Geometry: final body of the model. Coordinates: model frame, mm. Face numbers are marked on the shaded views. Round coordinates to 2 decimals unless told otherwise and drop trailing zeros. Order: outer loops, then holes, each group sorted by start corner. A loop starts at its lowest first (then second) coordinate and runs counter-clockwise, first axis right, second up. Notation, with made-up numbers: (19, 12.5) -> (48, 12.5) arc R9 ccw to (48, 18.5) -> close; hole circle Ø6 at (85, -13.75). An arc over 180 degrees is marked (long way). Put each result on its own line as item: value.
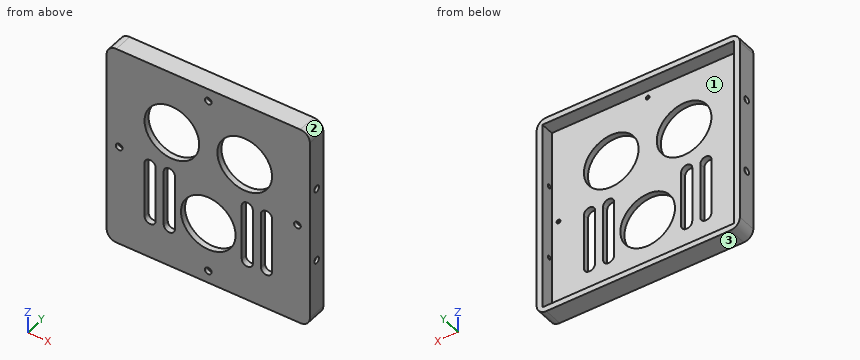
```python
from build123d import *

# Parameters (mm, degrees)
SKETCH1_W           = 106
SKETCH1_H           = 106
BOSS_EXTRUDE1_DEPTH = 10
SKETCH3_W           = 100
SKETCH3_H           = 100
CUT_EXTRUDE5_DEPTH  = 7
SKETCH7_R           = 14.25
CUT_EXTRUDE6_DEPTH  = 7
SKETCH9_R           = 1.75
CUT_EXTRUDE7_DEPTH  = 2
SKETCH11_R          = 1
CUT_EXTRUDE8_DEPTH  = 17
CUT_EXTRUDE9_DEPTH  = 1.5
SKETCH14_R          = 1
CUT_EXTRUDE10_DEPTH = 115.5
CUT_EXTRUDE11_START = -1.5
SKETCH15_R          = 1.75
CUT_EXTRUDE11_DEPTH = 1.5
FILLET1_R           = 5
CUT_EXTRUDE12_DEPTH = 10


with BuildPart() as part:
    # Sketch1 → Boss-Extrude1 (new body)
    with BuildSketch(Plane(origin=(0, 0, 0), x_dir=(1, 0, 0), z_dir=(0, 1, 0))):
        Rectangle(SKETCH1_W, SKETCH1_H)
    extrude(amount=BOSS_EXTRUDE1_DEPTH)

    # Sketch3 → Cut-Extrude5 (cut)
    with BuildSketch(Plane(origin=(0, 10, 0), x_dir=(1, 0, 0), z_dir=(0, 1, 0))):
        Rectangle(SKETCH3_W, SKETCH3_H)
    extrude(amount=-CUT_EXTRUDE5_DEPTH, mode=Mode.SUBTRACT)

    # Sketch7 → Cut-Extrude6 (cut)
    with BuildSketch(Plane(origin=(0, 3, 0), x_dir=(1, 0, 0), z_dir=(0, 1, 0))):
        with Locations(Location((0, 20.5, 0), (0, 0, 270))):
            Circle(SKETCH7_R)
        with Locations(Location((19, -20.5, 0), (0, 0, 270))):
            Circle(SKETCH7_R)
        with Locations(Location((-19, -20.5, 0), (0, 0, 270))):
            Circle(SKETCH7_R)
    extrude(amount=-CUT_EXTRUDE6_DEPTH, mode=Mode.SUBTRACT)

    # Sketch9 → Cut-Extrude7 (cut)
    with BuildSketch(Plane.XZ):
        with Locations(Location((46.5, 0, 0), (0, 0, 270))):
            Circle(SKETCH9_R)
        with Locations(Location((0, -46.5, 0), (0, 0, 270))):
            Circle(SKETCH9_R)
        with Locations(Location((0, 46.5, 0), (0, 0, 270))):
            Circle(SKETCH9_R)
        with Locations(Location((-46.5, 0, 0), (0, 0, 270))):
            Circle(SKETCH9_R)
    extrude(amount=-CUT_EXTRUDE7_DEPTH, mode=Mode.SUBTRACT)

    # Sketch11 → Cut-Extrude8 (cut)
    with BuildSketch(Plane.XZ.offset(-2)):
        with Locations(Location((46.5, 0, 0), (0, 0, 270))):
            Circle(SKETCH11_R)
        with Locations(Location((0, -46.5, 0), (0, 0, 270))):
            Circle(SKETCH11_R)
        with Locations(Location((-46.5, 0, 0), (0, 0, 270))):
            Circle(SKETCH11_R)
        with Locations(Location((0, 46.5, 0), (0, 0, 270))):
            Circle(SKETCH11_R)
    extrude(amount=-CUT_EXTRUDE8_DEPTH, mode=Mode.SUBTRACT)

    # Sketch12 → Cut-Extrude9 (cut)
    with BuildSketch(Plane(origin=(53, 0, 0), x_dir=(0, 0, -1), z_dir=(1, 0, 0))):
        with BuildLine():
            ThreePointArc((-17.75, 5), (-18.262563133, 6.237436867), (-19.5, 6.75))
            Line((-19.5, 6.75), (-19.5, 3.25))
            ThreePointArc((-19.5, 3.25), (-18.262563133, 3.762563133), (-17.75, 5))
        make_face()
        with BuildLine():
            Line((-19.5, 3.25), (-19.5, 6.75))
            ThreePointArc((-19.5, 6.75), (-21.25, 5), (-19.5, 3.25))
        make_face()
        with BuildLine():
            ThreePointArc((21.25, 5), (20.737436867, 6.237436867), (19.5, 6.75))
            Line((19.5, 6.75), (19.5, 3.25))
            ThreePointArc((19.5, 3.25), (20.737436867, 3.762563133), (21.25, 5))
        make_face()
        with BuildLine():
            Line((19.5, 3.25), (19.5, 6.75))
            ThreePointArc((19.5, 6.75), (17.75, 5), (19.5, 3.25))
        make_face()
    extrude(amount=-CUT_EXTRUDE9_DEPTH, mode=Mode.SUBTRACT)

    # Sketch14 → Cut-Extrude10 (cut)
    with BuildSketch(Plane(origin=(51.5, 0, 0), x_dir=(0, 0, -1), z_dir=(1, 0, 0))):
        with Locations((-19.5, 5)):
            Circle(SKETCH14_R)
        with Locations((19.5, 5)):
            Circle(SKETCH14_R)
    extrude(amount=-CUT_EXTRUDE10_DEPTH, mode=Mode.SUBTRACT)

    # Sketch15 → Cut-Extrude11 (cut)
    with BuildSketch(Plane.ZY.offset(53).offset(CUT_EXTRUDE11_START)):
        with Locations(Location((-19.5, 5, 0), (0, 0, 180))):
            Circle(SKETCH15_R)
        with Locations(Location((19.5, 5, 0), (0, 0, 180))):
            Circle(SKETCH15_R)
    extrude(amount=CUT_EXTRUDE11_DEPTH, mode=Mode.SUBTRACT)

    # Fillet1
    fillet1_edges = [part.edges().sort_by_distance(p)[0] for p in [
        (53, 5, 53),
        (-53, 5, 53),
        (-53, 5, -53),
        (53, 5, -53),
    ]]
    fillet(fillet1_edges, radius=FILLET1_R)

    # Sketch21 → Cut-Extrude12 (cut)
    with BuildSketch(Plane.XZ):
        with BuildLine():
            Line((-33.25, -31.84554788), (-33.25, -2.65445212))
            ThreePointArc((-33.25, -2.65445212), (-30.34554788, 0.25), (-27.441095759, -2.65445212))
            Line((-27.441095759, -2.65445212), (-27.441095759, -31.84554788))
            ThreePointArc((-27.441095759, -31.84554788), (-30.34554788, -34.75), (-33.25, -31.84554788))
        make_face()
        with BuildLine():
            Line((-23.25, -31.84554788), (-23.25, -2.65445212))
            ThreePointArc((-23.25, -2.65445212), (-20.34554788, 0.25), (-17.441095759, -2.65445212))
            Line((-17.441095759, -2.65445212), (-17.441095759, -31.84554788))
            ThreePointArc((-17.441095759, -31.84554788), (-20.34554788, -34.75), (-23.25, -31.84554788))
        make_face()
        with BuildLine():
            ThreePointArc((33.25, -31.84554788), (30.34554788, -34.75), (27.441095759, -31.84554788))
            Line((27.441095759, -31.84554788), (27.441095759, -2.65445212))
            ThreePointArc((27.441095759, -2.65445212), (30.34554788, 0.25), (33.25, -2.65445212))
            Line((33.25, -2.65445212), (33.25, -31.84554788))
        make_face()
        with BuildLine():
            Line((23.25, -31.84554788), (23.25, -2.65445212))
            ThreePointArc((23.25, -2.65445212), (20.34554788, 0.25), (17.441095759, -2.65445212))
            Line((17.441095759, -2.65445212), (17.441095759, -31.84554788))
            ThreePointArc((17.441095759, -31.84554788), (20.34554788, -34.75), (23.25, -31.84554788))
        make_face()
    extrude(amount=-CUT_EXTRUDE12_DEPTH, mode=Mode.SUBTRACT)


solid = part.part
```
1. Cut plane B-B on x = -30. Return loops of the section in (y, z), and give its area (3 significant figures).
Ans:
outline: (0, -53) -> (10, -53) -> (10, -50) -> (3, -50) -> (3, -34.73) -> (0, -34.73) -> close; (0, 0.23) -> (3, 0.23) -> (3, 11.44) -> (0, 11.44) -> close; (0, 29.56) -> (3, 29.56) -> (3, 50) -> (10, 50) -> (10, 53) -> (0, 53) -> close
area: 201 mm²
2. Cut plane A-A on z = 16. Return loops of the section in (x, y), and give its area (3 significant figures).
Ans:
outline: (-53, 0) -> (-32.52, 0) -> (-32.52, 3) -> (-50, 3) -> (-50, 10) -> (-53, 10) -> close; (-5.48, 0) -> (5.48, 0) -> (5.48, 3) -> (-5.48, 3) -> close; (32.52, 0) -> (53, 0) -> (53, 10) -> (50, 10) -> (50, 3) -> (32.52, 3) -> close
area: 198 mm²
3. Cut plane D-D on x = 39. Return loops of the section in (y, z).
Ans:
outline: (0, -53) -> (10, -53) -> (10, -50) -> (3, -50) -> (3, 50) -> (10, 50) -> (10, 53) -> (0, 53) -> close
4. Draft query along Z for the marked faces 1, 2 and 3. Return one class per face: +Z half, -Z half, draft (parallel to the pull), parting line (faces both ways), or undercut.
Ans:
face 1: undercut
face 2: +Z half
face 3: -Z half
5. Cut plane C-C on z = -38. Return loops of the section in (x, y), and give its area (3 significant figures).
Ans:
outline: (-53, 0) -> (53, 0) -> (53, 10) -> (50, 10) -> (50, 3) -> (-50, 3) -> (-50, 10) -> (-53, 10) -> close
area: 360 mm²
6. Material intervals for probe 1 along Z at (x, y) = (12, 8.5); probe 2 along X at (y, z) = (1, 20), sorted ascending.
Ans:
probe 1: -53 to -50, 50 to 53
probe 2: -53 to -33.24, -4.76 to 4.76, 33.24 to 53
7. Contact query for flat-ended pins moving along their axis: P1, Ø17, axis at x = 19, z = 20.5, coming from the +Y side; P2, Ø2.5, axis at x = 0, z = 46.5, coming from the +Y side; P3, Ø3, axis at y = 5, z = 19.5, coming from the +X side; P4, Ø3, axis at y = 5, z = 19.5, coming from the -X side. Output: stop coordinate, or through.
Ans:
P1: through
P2: y = 3
P3: x = 51.5
P4: x = -51.5
